Can you work these out from the drawing? Everything is in mm from the part's minimum corner. A direction names the side the tool comes from. Give positions to 0.01 mm unless a question says otherwise; leave off trailing zeros. Write each loop counter-clockwise with the first axis right and the second up, starting at its lowest first coordinate (ties: lowest second). Pieces come first, ordered by that corner, then holes. Notation, with made-up numbers: (9, -21) - (38, -21) arc R21 cw to (38, 10) - close; hole circle Ø2 at (55.25, -24.5). An arc over 180 degrees is marked (long way). Answer in a Markdown table with one row per item.
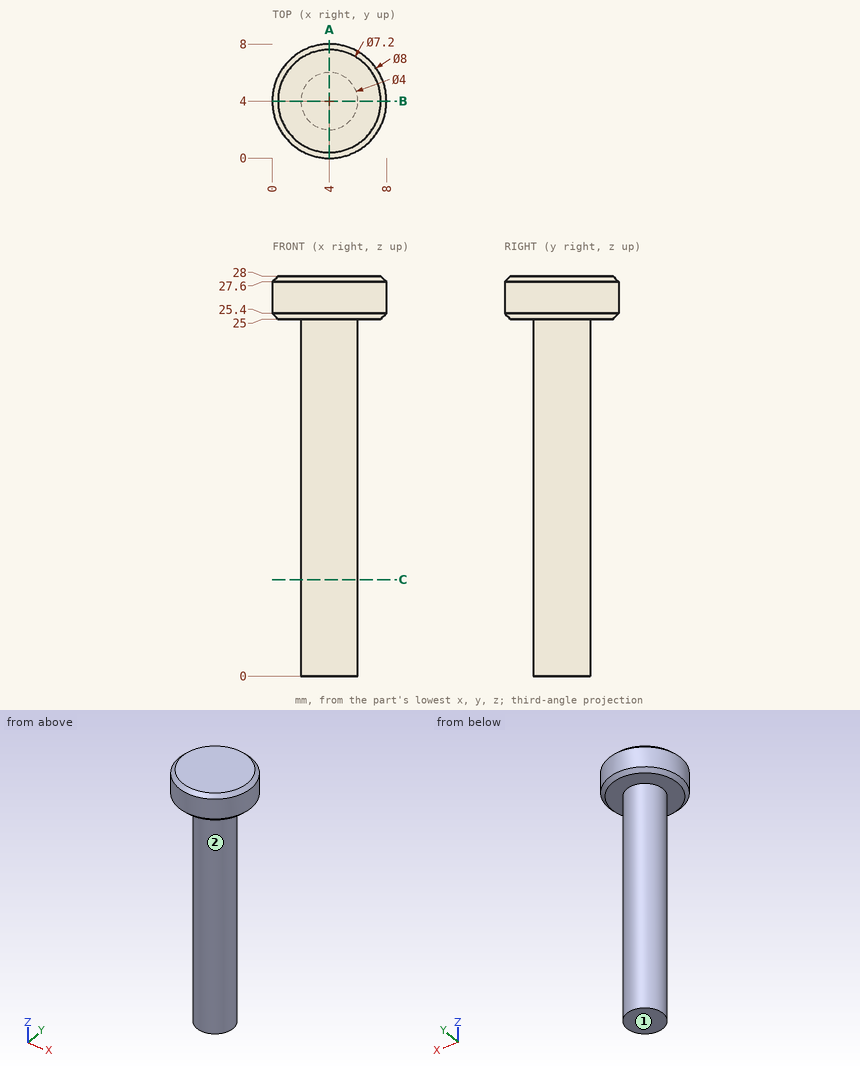
1) Imagine slicing it at C-C (z = 6.75). List the corners of the cut face in (x, y) for me, then the cut area to 3 significant figures.
Check values:
| item | result |
|---|---|
| outline | circle Ø4 at (4, 4) |
| area | 12.6 mm2 |
2) Imagine slicing it at A-A (x = 4). List the corners of the cut face in (y, z) for me.
Check values:
| item | result |
|---|---|
| outline | (0, 25.4) - (0.4, 25) - (2, 25) - (2, 0) - (6, 0) - (6, 25) - (7.6, 25) - (8, 25.4) - (8, 27.6) - (7.6, 28) - (0.4, 28) - (0, 27.6) - close |
3) On a 3-axis mill with a long thin cutter (end or side, diameter ignored), from which of +Z, -Z, +X, -X, +Y, -Y can I reach the whole of each face in a straight line? I mean the marked faces 1 and 2. Say none if no direction works.
Check values:
| item | result |
|---|---|
| face 1 | -Z, +X, -X, +Y, -Y |
| face 2 | -Z |
4) If I drill on line 1 (Y direction, x = 4, z = 7.5); line 2 (Z direction, x = 7.5, y = 4.5); line 3 (Y direction, x = 3, z = 10.5), over which ranges is the centre line in solid material (lowest first)?
Check values:
| item | result |
|---|---|
| line 1 | y = 2 to 6 |
| line 2 | z = 25 to 28 |
| line 3 | y = 2.27 to 5.73 |
5) Will these pins go through, and if not, where does the flat tip stop? P1, Ø2, axis at x = 5, y = 2.5, coming from the -Z side; P2, Ø1.5, axis at x = 2, z = 7, coming from the +Y side.
Check values:
| item | result |
|---|---|
| P1 | stops at z = 0 |
| P2 | stops at y = 5.56 |
